Geometry: see drawing. Coordinates: mm, zero at the bounding-box minimum. A direction names the side the tool comes from. Coordinates: 2 decimals unless noted, no trailing zeros. Loops run counter-clockwise (first coordinate to the right, second up) from the corner with the lowest first, then second, coordinate; pieces in that order, holes last. Notation, with made-up numbers: (-5.5, 37.25) -> (9.5, 37.25) arc R20 ccw to (9.5, 64.25) -> close; hole circle Ø4 at (32.25, -39.75). An arc over 180 degrees is marked (long way). Answer as a JSON object with one key per item and string values.
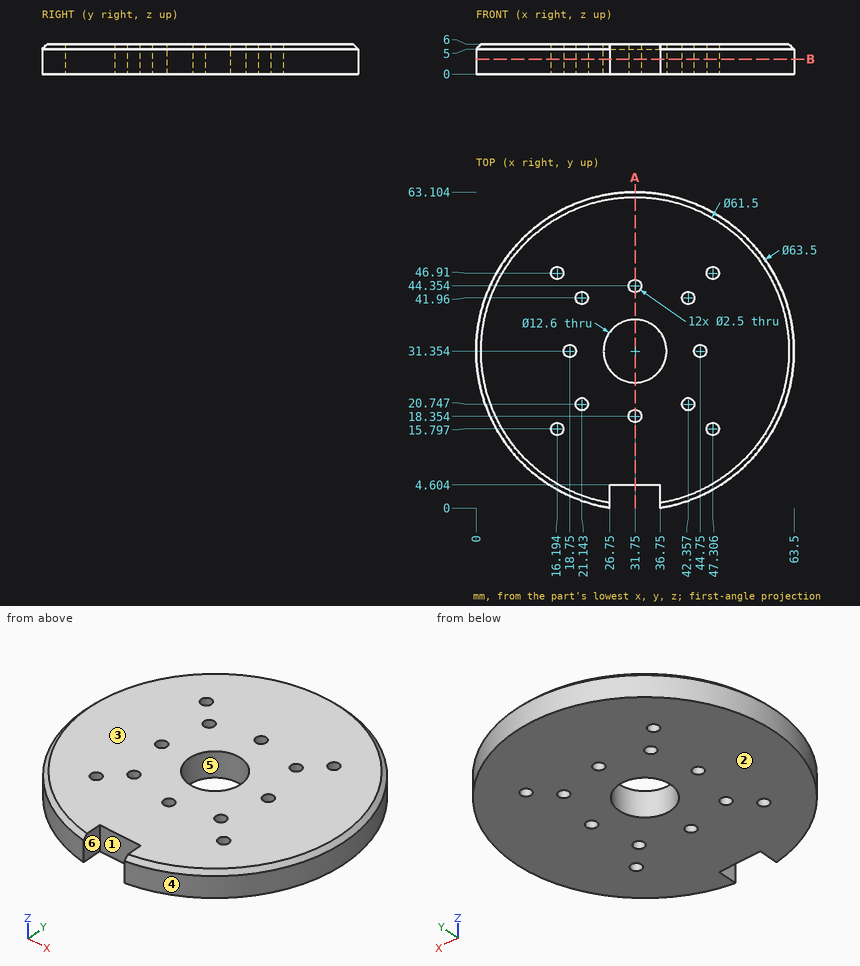
1. Access query for the marked faces 1 and 2. Directions: +Z, -Z, +X, -X, +Y, -Y. A direction counts if a zero-diameter tool reaches every point of the face in a straight line with its end or side. Return the directions, or none.
Reply:
{"face 1": "+Z, -Z, -Y", "face 2": "-Z, +X, -X, +Y, -Y"}
2. Line query: line 1 along X through (y, z) = (31.5, 5.5); line 2 along Y through (x, z) = (20.5, 1.5) (1 decimal); line 3 along X through (y, z) = (42, 3.5) (1 decimal). Output: solid intervals per line, ascending.
Reply:
{"line 1": "x = 0.5 to 17.51, 19.99 to 25.45, 38.05 to 43.51, 45.99 to 63", "line 2": "y = 1.7 to 19.7, 21.8 to 40.9, 43 to 61", "line 3": "x = 1.8 to 19.9, 22.4 to 41.1, 43.6 to 61.7"}
3. Section query A-A (x = 31.75). Return loops of the section in (y, z).
Reply:
{"outline": "(4.6, 0) -> (17.1, 0) -> (17.1, 6) -> (4.6, 6) -> close; (19.6, 0) -> (25.05, 0) -> (25.05, 6) -> (19.6, 6) -> close; (37.65, 0) -> (43.1, 0) -> (43.1, 6) -> (37.65, 6) -> close; (45.6, 0) -> (63.1, 0) -> (63.1, 5) -> (62.1, 6) -> (45.6, 6) -> close"}
4. Pin query (flat end, axial travel): P1, Ø1.4, axis at y = 3, z = 2.5, coming from the +X side; P2, Ø3, axis at y = 30, z = 2, coming from the -X side; P3, Ø3, axis at x = 30.5, z = 4, coming from the -Y side; P4, Ø2.5, axis at y = 1.5, z = 3.5, coming from the -X side. Return the tip coordinate at first contact, or that it passes through.
Reply:
{"P1": "stops at x = 47.35", "P2": "stops at x = 0", "P3": "stops at y = 4.6", "P4": "stops at x = 17.97"}
5. Section query B-B (z = 3). Count the separate pieces of the cut face and the enclosed holes in it, plus the area to 3 significant figures.
Reply:
{"separate pieces": "1", "enclosed holes": "13", "area": "2,930 mm2"}
6. Mould query, pull axis X, two halves, no side actions, for the marked faces 3, 4, 5 and 6. Classes: pulls with the +X half, pulls with the -X half, needs draft (parallel to the pull), parting line crosses it, or undercut.
Reply:
{"face 3": "needs draft", "face 4": "parting line crosses it", "face 5": "undercut", "face 6": "undercut"}
